Autodesk Inventor part; units mm, degrees
ref_plane "YZ Plane" through (0, 0, 0) normal (1, 0, 0) x (0, 1, 0)
ref_plane "XZ Plane" through (0, 0, 0) normal (0, 1, 0) x (-1, 0, 0)
ref_plane "XY Plane" through (0, 0, 0) normal (0, 0, 1) x (1, 0, 0)
sketch "Sketch1" plane through (0, 0, 0) normal (0, 1, 0) x (-1, 0, 0)
  line L0 (35.56, 50.8) -> (-35.56, 50.8)
  line L1 (-35.56, 50.8) -> (-35.56, -50.8)
  line L2 (-35.56, -50.8) -> (35.56, -50.8)
  line L3 (35.56, -50.8) -> (35.56, 50.8)
  point P0 (0, 0)
  point P1 (35.56, 0)
  point P2 (0, -50.8)
  dimension "d0" = 101.6
  dimension "d1" = 71.12
extrude "Extrusion1" add sketch "Sketch1" along normal blind 2
sketch "Sketch2" plane through (0, 2, 0) normal (0, 1, 0) x (1, 0, 0)
  line L0 (-35.56, 50.8) -> (-35.56, -50.8)
  line L1 (35.56, 50.8) -> (-35.56, 50.8)
  line L2 (35.56, -50.8) -> (35.56, 50.8)
  line L3 (-35.56, -50.8) -> (35.56, -50.8)
  point P0 (0, 0)
  point P1 (-10.16, -35.56)
  point P2 (-29.21, 44.45)
  point P3 (29.21, 44.45)
  point P4 (29.21, -44.45)
  dimension "d4" = 6.35
  dimension "d5" = 6.35
  dimension "d6" = 6.35
  dimension "d7" = 6.35
  dimension "d8" = 15.24
  dimension "d9" = 45.72
hole "Hole1" at (-10.16, 2, 35.56) at (-29.21, 2, -44.45) at (29.21, 2, -44.45) at (29.21, 2, 44.45) direction (0, -1, 0) diameter 3.1999 end through all
sketch "Sketch3" plane through (0, 2, 0) normal (0, 1, 0) x (1, 0, 0)
  line L0 (-32.412, -43.7017) -> (-16.972, -43.7017)
  line L1 (-16.972, -43.7017) -> (-16.972, 4.5583)
  line L2 (-16.972, 4.5583) -> (-32.412, 4.5583)
  line L3 (-32.412, 4.5583) -> (-32.412, -43.7017)
  line L4 (-35.56, -50.8) -> (35.56, -50.8)
  line L5 (-35.56, 50.8) -> (-35.56, -50.8)
  point P0 (0, 0)
  dimension "d17" = 15.44
  dimension "d18" = 48.26
  dimension "d19" = 7.0983
  dimension "d20" = 3.148
extrude "Extrusion2" add sketch "Sketch3" along normal blind 5.08
sketch "Sketch4" plane through (0, 2, 0) normal (0, 1, 0) x (1, 0, 0)
  line L0 (-34.03, 11.2383) -> (-21.03, 11.2383)
  line L1 (-21.03, 11.2383) -> (-21.03, 20.7383)
  line L2 (-21.03, 20.7383) -> (-34.03, 20.7383)
  line L3 (-34.03, 20.7383) -> (-34.03, 11.2383)
  line L4 (-34.03, 24.6583) -> (-19.81, 24.6583)
  line L5 (-19.81, 24.6583) -> (-19.81, 34.8183)
  line L6 (-19.81, 34.8183) -> (-34.03, 34.8183)
  line L7 (-34.03, 34.8183) -> (-34.03, 24.6583)
  line L8 (-14.98, 36.27) -> (-5.48, 36.27)
  line L9 (-5.48, 36.27) -> (-5.48, 49.27)
  line L10 (-5.48, 49.27) -> (-14.98, 49.27)
  line L11 (-14.98, 49.27) -> (-14.98, 36.27)
  line L12 (-16.972, 4.5583) -> (-32.412, 4.5583)
  line L13 (-35.56, 50.8) -> (-35.56, -50.8)
  line L14 (35.56, 50.8) -> (-35.56, 50.8)
  point P0 (0, 0)
  dimension "d23" = 13
  dimension "d24" = 9.5
  dimension "d25" = 3.92
  dimension "d26" = 6.68
  dimension "d27" = 1.53
  dimension "d28" = 1.53
  dimension "d29" = 20.58
  dimension "d66" = 14.22
  dimension "d67" = 13
  dimension "d68" = 10.16
extrude "Extrusion3" add sketch "Sketch4" along normal blind 10
sketch "Sketch5" plane through (0, 2, 0) normal (0, 1, 0) x (1, 0, 0)
  line L0 (3.1628, -21.8228) -> (19.1628, -21.8228)
  line L1 (19.1628, -21.8228) -> (19.1628, -4.6228)
  line L2 (19.1628, -4.6228) -> (3.1628, -4.6228)
  line L3 (3.1628, -4.6228) -> (3.1628, -21.8228)
  line L4 (3.1628, 11.7072) -> (19.1628, 11.7072)
  line L5 (19.1628, 11.7072) -> (19.1628, 28.9072)
  line L6 (19.1628, 28.9072) -> (3.1628, 28.9072)
  line L7 (3.1628, 28.9072) -> (3.1628, 11.7072)
  line L8 (35.56, -50.8) -> (35.56, 50.8)
  line L9 (35.56, 50.8) -> (-35.56, 50.8)
  point P0 (0, 0)
  dimension "d32" = 17.2
  dimension "d33" = 16
  dimension "d34" = 16.33
  dimension "d35" = 16.3972
  dimension "d36" = 21.8928
extrude "Extrusion4" add sketch "Sketch5" along normal blind 3
sketch "Sketch6" plane through (0, 2, 0) normal (0, 1, 0) x (1, 0, 0)
  circle A0 centre (6.61, -27.94) radius 3.75
  circle A1 centre (6.61, 5.58) radius 3.75
  line L0 (35.56, -50.8) -> (35.56, 50.8)
  line L1 (-35.56, -50.8) -> (35.56, -50.8)
  point P0 (0, 0)
  dimension "d39" = 7.5
  dimension "d40" = 26.02
  dimension "d41" = 25.2
  dimension "d42" = 19.11
extrude "Extrusion5" add sketch "Sketch6" along normal blind 6.35
sketch "Sketch7" plane through (0, 2, 0) normal (0, 1, 0) x (1, 0, 0)
  line L0 (11.4397, -48.5168) -> (13.9664, -48.5168)
  line L1 (13.9664, -48.5168) -> (13.9664, -40.9016)
  line L2 (13.9664, -40.9016) -> (11.4397, -40.9016)
  line L3 (11.4397, -40.9016) -> (11.4397, -48.5168)
  line L4 (14.4877, -48.5168) -> (17.0144, -48.5168)
  line L5 (17.0144, -48.5168) -> (17.0144, -40.9016)
  line L6 (17.0144, -40.9016) -> (14.4877, -40.9016)
  line L7 (14.4877, -40.9016) -> (14.4877, -48.5168)
  line L8 (17.5357, -48.5168) -> (20.0624, -48.5168)
  line L9 (20.0624, -48.5168) -> (20.0624, -40.9016)
  line L10 (20.0624, -40.9016) -> (17.5357, -40.9016)
  line L11 (17.5357, -40.9016) -> (17.5357, -48.5168)
  line L12 (20.5837, -48.5168) -> (23.1104, -48.5168)
  line L13 (23.1104, -48.5168) -> (23.1104, -40.9016)
  line L14 (23.1104, -40.9016) -> (20.5837, -40.9016)
  line L15 (20.5837, -40.9016) -> (20.5837, -48.5168)
  line L16 (28.7104, -27.1717) -> (31.2273, -27.1717)
  line L17 (31.2273, -27.1717) -> (31.2273, -11.9647)
  line L18 (31.2273, -11.9647) -> (28.7104, -11.9647)
  line L19 (28.7104, -11.9647) -> (28.7104, -27.1717)
  line L20 (31.7584, -27.1717) -> (34.2753, -27.1717)
  line L21 (34.2753, -27.1717) -> (34.2753, -11.9647)
  line L22 (34.2753, -11.9647) -> (31.7584, -11.9647)
  line L23 (31.7584, -11.9647) -> (31.7584, -27.1717)
  line L24 (28.7104, 6.3564) -> (31.2273, 6.3564)
  line L25 (31.2273, 6.3564) -> (31.2273, 21.5633)
  line L26 (31.2273, 21.5633) -> (28.7104, 21.5633)
  line L27 (28.7104, 21.5633) -> (28.7104, 6.3564)
  line L28 (-35.56, -50.8) -> (35.56, -50.8)
  line L29 (-8.89, -45.974) -> (8.89, -45.974)
  line L30 (8.89, -45.974) -> (8.89, -40.894)
  line L31 (8.89, -40.894) -> (-8.89, -40.894)
  line L32 (-8.89, -40.894) -> (-8.89, -45.974)
  line L33 (35.56, -50.8) -> (35.56, 50.8)
  line L34 (31.7584, 6.3564) -> (34.2753, 6.3564)
  line L35 (34.2753, 6.3564) -> (34.2753, 21.5633)
  line L36 (34.2753, 21.5633) -> (31.7584, 21.5633)
  line L37 (31.7584, 21.5633) -> (31.7584, 6.3564)
  line L38 (35.56, 50.8) -> (-35.56, 50.8)
  point P0 (0, 0)
  dimension "d47" = 7.6152
  dimension "d48" = 4.826
  dimension "d49" = 5.08
  dimension "d50" = 2.2832
  dimension "d51" = 2.5268
  dimension "d52" = 0.5212
  dimension "d53" = 0.5212
  dimension "d54" = 0.5212
  dimension "d55" = 12.4496
  dimension "d56" = 2.5497
  dimension "d57" = 17.78
  dimension "d58" = 15.207
  dimension "d59" = 2.5169
  dimension "d60" = 0.5311
  dimension "d61" = 18.321
  dimension "d62" = 1.2847
  dimension "d63" = 29.2367
extrude "Extrusion6" add sketch "Sketch7" along normal blind 2
equation "\"d67\" = d23"
equation "\"d53\" = d52"
equation "\"d54\" = d52"
properties part number "PCB"
Input: part model. Units: mm. Frame: model coordinates. A direction names the side the tool comes from. Give positions to 0.01 mm unless a question says otherwise; leave off trailing zeros. Loops run counter-clockwise (first coordinate to the right, second up) from the corner with the lowest first, then second, coordinate; pieces in that order, holes last. Notation, with made-up numbers: (84, 89.5) - (129, 89.5) arc R25 ccw to (129, 115.5) - close; hole circle Ø10 at (59, 47). An arc over 180 degrees is marked (long way). Use CSV: the item, a comma, the result in double quotes. Start each with the question number.
Item 1: Section B-B on z = 35.56. Return loops of the section in (x, y).
Item 2: Mould query, pull axis X, two halves, no side actions, for faces 1 (the flat face through (13, 3, 48.517)), 2 (the flat face through (-35.56, 1, -1)), 3 (the flat face through (31.758, 3, -14)), 4 (the flat face through (17.014, 3, 45)). Classes: pulls with the +X half, pulls with the -X half, needs draft (parallel to the pull), parting line crosses it, or undercut.
Item 3: Section D-D on x = 6.61. Return loops of the section in (y, z), then the cut area to 3 significant figures.
Item 4: Line query: line 1 (X direction, y = 1.1, z = -44.45); line 2 (Z direction, x = 12, y = 3.5); line 3 (X direction, y = 1.45, z = 35.56). Output: solid intervals per line, ascending.
Item 5: Contact query for flat-ended pins moving along their axis: P1, Ø2, axis at x = 18.5, z = 46.5, coming from the +Y side; P2, Ø1.6, axis at y = 3.5, z = -12, coming from the +X side; P3, Ø4, axis at x = -7, z = 17, coming from the -Y side; P4, Ø0.6, axis at y = 2.5, z = 45, coming from the +X side. Output: stop coordinate, or through.
Item 6: Reachability of faces 5 (the flat face through (13.966, 3, 45)), 6 (the flat face through (19, 4, 45)), 7 (the flat face through (11, 3, -11.707)), 8 (the flat face through (19.163, 3, 13)), 9 (the flat face through (33, 3, -21.563)) from +Z, -Z, +X, -X, +Y, -Y: full face, straight path, thin tool, end or side. Return the list, or none.
Item 7: Section C-C on z = 6.5. Return loops of the section in (x, y), then the cut area to 3 significant figures.
Item 8: Section A-A on x = -10.16. Return loops of the section in (y, z).
Ans:
1,outline,"(-35.56, 0) - (-11.76, 0) - (-11.76, 2) - (-16.97, 2) - (-16.97, 7.08) - (-32.41, 7.08) - (-32.41, 2) - (-35.56, 2) - close; (-8.56, 0) - (35.56, 0) - (35.56, 2) - (-8.56, 2) - close"
2,face 1,"needs draft"
2,face 2,"pulls with the -X half"
2,face 3,"undercut"
2,face 4,"undercut"
3,outline,"(0, -50.8) - (2, -50.8) - (2, -28.91) - (5, -28.91) - (5, -11.71) - (2, -11.71) - (2, -9.33) - (8.35, -9.33) - (8.35, -1.83) - (2, -1.83) - (2, 4.62) - (5, 4.62) - (5, 21.82) - (2, 21.82) - (2, 24.19) - (8.35, 24.19) - (8.35, 31.69) - (2, 31.69) - (2, 40.89) - (4, 40.89) - (4, 45.97) - (2, 45.97) - (2, 50.8) - (0, 50.8) - close"
3,area,"412 mm2"
4,line 1,"x = -35.56 to -30.81, -27.61 to 27.61, 30.81 to 35.56"
4,line 2,"z = -28.91 to -11.71, 4.62 to 21.82, 40.9 to 48.52"
4,line 3,"x = -35.56 to -11.76, -8.56 to 35.56"
5,P1,"stops at y = 4"
5,P2,"stops at x = 34.28"
5,P3,"stops at y = 0"
5,P4,"stops at x = 23.11"
6,face 5,"+Z, +Y"
6,face 6,"+Z, +X, +Y"
6,face 7,"+Y"
6,face 8,"-Z, +Y"
6,face 9,"-Z, +X, +Y"
7,outline,"(-35.56, 0) - (35.56, 0) - (35.56, 2) - (19.16, 2) - (19.16, 5) - (3.16, 5) - (3.16, 2) - (-16.97, 2) - (-16.97, 7.08) - (-32.41, 7.08) - (-32.41, 2) - (-35.56, 2) - close"
7,area,"269 mm2"
8,outline,"(0, -50.8) - (2, -50.8) - (2, -49.27) - (12, -49.27) - (12, -36.27) - (2, -36.27) - (2, 33.96) - (0, 33.96) - close; (0, 37.16) - (2, 37.16) - (2, 50.8) - (0, 50.8) - close"
